```python
from build123d import *

# Parameters (mm, degrees)
SKETCH1_R               = 4.826
SKETCH1_R_2             = 3.429
BOSS_EXTRUDE1_DEPTH     = 12.7
SKETCH2_R               = 3.429
SKETCH2_R_2             = 1.905
BOSS_EXTRUDE2_DEPTH     = 6.35
BOSS_EXTRUDE4_DEPTH     = 6.35
CUT_EXTRUDE1_DEPTH      = 7.35
CUT_EXTRUDE1_DEPTH_BACK = 7.35
SKETCH6_R               = 1.778
CUT_EXTRUDE2_DEPTH      = 6.35


with BuildPart() as part:
    # Sketch1 → Boss-Extrude1 (new body)
    with BuildSketch(Plane(origin=(0, 0, 0), x_dir=(1, 0, 0), z_dir=(0, 1, 0))):
        with BuildLine():
            Line((-9.906, 6.35), (9.906, 6.35))
            ThreePointArc((9.906, 6.35), (16.256, 0), (9.906, -6.35))
            Line((9.906, -6.35), (-9.906, -6.35))
            ThreePointArc((-9.906, -6.35), (-16.256, 0), (-9.906, 6.35))
        make_face()
        Circle(SKETCH1_R, mode=Mode.SUBTRACT)
        with Locations((9.906, 0)):
            Circle(SKETCH1_R_2, mode=Mode.SUBTRACT)
        with Locations((-9.906, 0)):
            Circle(SKETCH1_R_2, mode=Mode.SUBTRACT)
    extrude(amount=BOSS_EXTRUDE1_DEPTH)

    # Sketch2 → Boss-Extrude2 (add)
    with BuildSketch(Plane(origin=(0, 0, 0), x_dir=(1, 0, 0), z_dir=(0, 1, 0))):
        with Locations((-9.906, 0)):
            Circle(SKETCH2_R)
        with Locations((-9.906, 0)):
            Circle(SKETCH2_R_2, mode=Mode.SUBTRACT)
        with Locations((9.906, 0)):
            Circle(SKETCH2_R)
        with Locations((9.906, 0)):
            Circle(SKETCH2_R_2, mode=Mode.SUBTRACT)
    extrude(amount=BOSS_EXTRUDE2_DEPTH)

    # Sketch4 → Boss-Extrude4 (add)
    with BuildSketch(Plane(origin=(0, 0, 0), x_dir=(1, 0, 0), z_dir=(0, 1, 0))):
        with BuildLine():
            ThreePointArc((-14.03301151, -4.826), (-15.67353947, -2.656687497), (-16.256, 0))
            Line((-16.256, 0), (-112.268, 0))
            Line((-112.268, 0), (-112.268, -4.826))
            Line((-112.268, -4.826), (-14.03301151, -4.826))
        make_face()
        with BuildLine():
            Line((-112.268, 0), (-16.256, 0))
            ThreePointArc((-16.256, 0), (-15.67353947, 2.656687497), (-14.03301151, 4.826))
            Line((-14.03301151, 4.826), (-112.268, 4.826))
            ThreePointArc((-112.268, 4.826), (-117.094, 0), (-112.268, -4.826))
            Line((-112.268, -4.826), (-112.268, 0))
        make_face()
    extrude(amount=BOSS_EXTRUDE4_DEPTH)

    # Sketch5 → Cut-Extrude1 (cut, two sides)
    with BuildSketch(Plane.XY) as cut_extrude1_sk:
        Polygon((-117.094, 6.35), (-16.110356901, 6.35), (-117.094, 3.175), align=None)
    extrude(amount=CUT_EXTRUDE1_DEPTH, mode=Mode.SUBTRACT)
    extrude(cut_extrude1_sk.sketch, amount=-CUT_EXTRUDE1_DEPTH_BACK, mode=Mode.SUBTRACT)

    # Sketch6 → Cut-Extrude2 (cut)
    with BuildSketch(Plane(origin=(0, 0, 0), x_dir=(1, 0, 0), z_dir=(0, 1, 0))):
        with Locations((-112.268, 0)):
            Circle(SKETCH6_R)
    extrude(amount=CUT_EXTRUDE2_DEPTH, mode=Mode.SUBTRACT)


solid = part.part
```
Model file for the job. Use its own axes, mm. A direction names the side the tool comes from. Give positions to 0.01 mm unless a question says otherwise; leave off trailing zeros. Loops run counter-clockwise (first coordinate to the right, second up) from the corner with the lowest first, then second, coordinate; pieces in that order, holes last. Notation, with made-up numbers: (72.5, -28.5) - (126.5, -28.5) arc R22 ccw to (126.5, 5.5) - close; hole circle Ø8 at (-39.75, 29). An arc over 180 degrees is marked (long way). One line per item, written item: value. Start each with the question number.
1. Slice it at A-A (x = 0). List the corners of the cut face in (y, z).
2. Slice it at D-D (x = -31.5). List the corners of the cut face in (y, z).
3. Which spindle directions (+Z, -Z, +X, -X, +Y, -Y) get a long thin tool onto all of the face, cutting with end or side? Do faces 5 (the flat face through (11.4, 6.35, 1.5)), 6 (the flat face through (-64, 2, 4.826)), 7 (the flat face through (-15.5, 6.35, -3.9)). Say none if no direction does.
4. Pin check, flat tips, straight feed: pin 1 (1.9 mm diameter, centred on x = -46.5, y = 4.5, fed in from -Z); pin 2 (4 mm diameter, centred on x = 9.906, z = 0, fed in from +Y); pin 3 (3 mm diameter, centred on x = -42.5, y = 4, fed in from +Z). Stop position of each tip, or through.
5. Probe L1, parallel to X at y = 8.5, z = 0 (3 decimals); L2, parallel to X at y = 2.25, z = 0; L3, parallel to X at y = 1.75, z = -1.25. List the from-to ranges inside material, lowest first. Write a range as from..to.
6. Pull direction Z, two halves, no side cores. Call faces 1 (the flat face through (0, 6, 6.35)), 2 (the cylindrical face through (16.254, 6.261, -0.14)), 3 (the cylindrical face through (-3.83, 6.261, 2.937)), 4 (the cylindrical face through (-13.33, 9.48, -0.15)): pulls with the +Z half, pulls with the -Z half, needs draft (parallel to the pull), parting line crosses it, or undercut.
7. Slice it at B-B (z = 0). Give the number of separate pieces and of enclosed holes in the cut face, plus the area to 3 significant figures.
8. Slice it at C-C (y = 8.75). List the corners of the cut face in (x, z) (3 decimals), plus the area to 3 significant figures.
Solution:
1. outline: (0, -6.35) - (12.7, -6.35) - (12.7, -4.83) - (0, -4.83) - close; (0, 4.83) - (12.7, 4.83) - (12.7, 6.35) - (0, 6.35) - close
2. outline: (0, -4.83) - (5.87, -4.83) - (5.87, 4.83) - (0, 4.83) - close
3. face 5: +Y
3. face 6: +Z, -X, +Y, -Y
3. face 7: -Z, -X, +Y
4. pin 1: stops at z = -4.83
4. pin 2: stops at y = 6.35
4. pin 3: stops at z = 4.83
5. L1: x = -16.256..-13.335, -6.477..-4.826, 4.826..6.477, 13.335..16.256
5. L2: x = -117.09..-114.05, -110.49..-11.81, -8..-4.83, 4.83..8, 11.81..16.26
5. L3: x = -116.93..-113.53, -111..-11.34, -8.47..-4.66, 4.66..8.47, 11.34..16.13
6. face 1: pulls with the +Z half
6. face 2: parting line crosses it
6. face 3: undercut
6. face 4: undercut
7. separate pieces: 5
7. enclosed holes: 0
7. area: 623 mm^2
8. outline: (-9.906, -6.35) - (9.906, -6.35) arc R6.35 ccw to (9.906, 6.35) - (-9.906, 6.35) arc R6.35 ccw to start; hole circle Ø6.858 at (-9.906, 0); hole circle Ø9.652 at (0, 0); hole circle Ø6.858 at (9.906, 0)
8. area: 231 mm^2
